Geometry: final body of the model. Coordinates: model frame, mm. A direction names the side the tool comes from. Round coordinates to 2 decimals unless told otherwise and drop trailing zeros. Loops run counter-clockwise (first coordinate to the right, second up) from the corner with the lowest first, then second, coordinate; pieces in that order, holes last. Notation, with made-up numbers: (87.5, -23) - (97.5, -23) arc R15 cw to (97.5, 5) - close; hole circle Ø9 at (-32.5, 0). An arc over 180 degrees is marked (long way). Answer as CSV lines item,"result".
from build123d import *

# Parameters (mm, degrees)
SKETCH2_W      = 8.226207469
SKETCH2_H      = 12.781412334
EXTRUDE1_DEPTH = 11.331323155
SKETCH6_W      = 0.508
SKETCH6_H      = 0.508
EXTRUDE2_DEPTH = 25.908
SKETCH7_W      = 0.508
SKETCH7_H      = 0.508


with BuildPart() as part:
    # Sketch1 → Revolve1 (revolve)
    with BuildSketch(Plane(origin=(0, 0, 0), x_dir=(0, 0, -1), z_dir=(1, 0, 0)), mode=Mode.PRIVATE) as revolve1_sk:
        with BuildLine():
            Line((0, 8.4074), (0, 0))
            Line((0, 0), (2.7813, 0))
            Line((2.7813, 0), (2.7813, 0.9144))
            Line((2.7813, 0.9144), (2.4765, 0.9144))
            Line((2.4765, 0.9144), (2.3876, 6.060688583))
            ThreePointArc((2.3876, 6.060688583), (1.67389428, 7.722503628), (0, 8.4074))
        make_face()
    revolve(revolve1_sk.sketch.rotate(Axis((0, 8.4074, 0), (0, -1, 0)), 180), axis=Axis((0, 8.4074, 0), (0, -1, 0)))

    # Sketch2 → Extrude1 (cut, through all)
    with BuildSketch(Plane.XY.offset(2.54)):
        with Locations((-0.622714808, 4.861343099)):
            Rectangle(SKETCH2_W, SKETCH2_H)
    extrude(amount=EXTRUDE1_DEPTH, mode=Mode.SUBTRACT)

    # Sketch6 → Extrude2 (add)
    with BuildSketch(Plane(origin=(0, 0, 0), x_dir=(1, 0, 0), z_dir=(0, 1, 0))):
        with Locations((0, -1.27)):
            Rectangle(SKETCH6_W, SKETCH6_H)
    extrude(amount=-EXTRUDE2_DEPTH)

    # Sweep1: sweep along a path in Sketch5
    with BuildLine(Plane(origin=(0, 0, 0), x_dir=(0, 0, -1), z_dir=(1, 0, 0))) as sweep1_path:
        Line((1.27, 0), (1.27, -5.69243597))
        ThreePointArc((1.27, -5.69243597), (1.390841242, -6.299945919), (1.734967985, -6.814967985))
        Line((1.734967985, -6.814967985), (8.425032015, -13.505032015))
        ThreePointArc((8.425032015, -13.505032015), (8.769158758, -14.020054081), (8.89, -14.62756403))
        Line((8.89, -14.62756403), (8.89, -25.908))
    # Sketch7 → Sweep1 (sweep)
    with BuildSketch(Plane(origin=(0, 0, 0), x_dir=(1, 0, 0), z_dir=(0, 1, 0))):
        with Locations((0, 1.27)):
            Rectangle(SKETCH7_W, SKETCH7_H)
    sweep(path=sweep1_path.line)


solid = part.part
(1) Access query for faces 1 (the face through (0, 0.5, 2.54)), 2 (the face through (-0.254, -12, -7)). Directions: +Z, -Z, +X, -X, +Y, -Y. A direction counts if a zero-diameter tool reaches every point of the face in a straight line with its end or side. Return the directions, or none.
Findings below:
face 1,"+Z, +X, -X, +Y, -Y"
face 2,"+Z, -Z, -X, -Y"
(2) Pin query (flat end, axial travel): P1, Ø1, axis at x = 0, y = 2, coming from the +Z side; P2, Ø2, axis at x = -1, z = -4, coming from the +Y side; P3, Ø1, axis at x = -1.5, z = 1.5, coming from the +Y side. Return the tip coordinate at first contact, or that it passes through.
Findings below:
P1,"z = 2.47"
P2,"y = -8.05"
P3,"y = 7.77"
(3) Section D-D (y = 3). Output: boundary loops of the cut face in (x, z).
Findings below:
outline,"circle Ø4.88 at (0, 0)"
(4) Section B-B (y = -12.5). Output: boundary loops of the cut face in (x, z), and give its area (3 significant figures).
Findings below:
outline,"(-0.25, -7.78) - (0.25, -7.78) - (0.25, -7.06) - (-0.25, -7.06) - close; (-0.25, 1.02) - (0.25, 1.02) - (0.25, 1.52) - (-0.25, 1.52) - close"
area,"0.623 mm2"
(5) Section A-A (y = -0.5). Output: boundary loops of the cut face in (x, z).
Findings below:
outline,"(-0.25, -1.52) - (0.25, -1.52) - (0.25, -1.02) - (-0.25, -1.02) - close; (-0.25, 1.02) - (0.25, 1.02) - (0.25, 1.52) - (-0.25, 1.52) - close"
(6) Material intervals for line 1 along Y through (x, z) = (-2.2, 1.5); line 2 along Y through (x, z) = (0.1, -1.75); line 3 along X through (y, z) = (-13, -8), sorted ascending.
Findings below:
line 1,"0 to 0.91"
line 2,"-7.19 to -6.44, 0 to 7.64"
line 3,"-0.25 to 0.25"
(7) Section C-C (z = -6.75). Output: boundary loops of the cut face in (x, y), and give its area (3 significant figures).
Findings below:
outline,"(-0.25, -12.19) - (0.25, -12.19) - (0.25, -11.47) - (-0.25, -11.47) - close"
area,"0.365 mm2"
(8) Draft query along Z for faces 3 (the face through (0.254, -12, -7)), 4 (the face through (-0.11, 3.52, -2.43)), 5 (the face through (0, -10.39, -4.95)). Return one class per face: pulls with the +Z half, pulls with the -Z half, needs draft (parallel to the pull), parting line crosses it, or undercut.
Findings below:
face 3,"needs draft"
face 4,"parting line crosses it"
face 5,"undercut"
